Design review of the part built by this model. Coordinates are the model's own, in mm. A direction names the side the tool comes from. Coordinates: 2 decimals unless noted, no trailing zeros. Loops run counter-clockwise (first coordinate to the right, second up) from the corner with the lowest first, then second, coordinate; pieces in that order, holes last. Notation, with made-up numbers: (57.5, 30) -> (99.5, 30) arc R14 cw to (99.5, 47) -> close; hole circle Ø5 at (17.25, -38.75). An arc over 180 degrees is marked (long way). Use CSV: the item, a comma, the result in double quotes.
```python
from build123d import *

# Parameters (mm, degrees)
F0_R     = 12.7
F1_DEPTH = 25.4


with BuildPart() as f1:
    # F0 (on Front) → F1 (new body)
    with BuildSketch(Plane.XZ):
        with BuildLine():
            Line((16.9537905604, 25.4), (-42.3537905604, 25.4))
            ThreePointArc((-42.3537905604, 25.4), (-24.3932783182, 17.9605122421), (-16.9537905604, 0))
            ThreePointArc((-16.9537905604, 0), (-24.3932783182, -17.9605122421), (-42.3537905604, -25.4))
            Line((-42.3537905604, -25.4), (16.9537905604, -25.4))
            ThreePointArc((16.9537905604, -25.4), (34.9143028025, -17.9605122421), (42.3537905604, 0))
            ThreePointArc((42.3537905604, 0), (34.9143028025, 17.9605122421), (16.9537905604, 25.4))
        make_face()
        with Locations((16.9537905604, 0)):
            Circle(F0_R, mode=Mode.SUBTRACT)
        with BuildLine():
            Line((-42.3537905604, 14.224), (-42.3537905604, 25.4))
            ThreePointArc((-42.3537905604, 25.4), (-67.7537905604, 0), (-42.3537905604, -25.4))
            Line((-42.3537905604, -25.4), (-42.3537905604, -14.224))
            ThreePointArc((-42.3537905604, -14.224), (-56.5777905604, 0), (-42.3537905604, 14.224))
        make_face()
        with BuildLine():
            ThreePointArc((-16.9537905604, 0), (-24.3932783182, 17.9605122421), (-42.3537905604, 25.4))
            Line((-42.3537905604, 25.4), (-42.3537905604, 14.224))
            ThreePointArc((-42.3537905604, 14.224), (-33.8234800273, 11.3822659523), (-28.7016163276, 3.9925323692))
            Line((-28.7016163276, 3.9925323692), (-23.993383965, 3.9925323692))
            Line((-23.993383965, 3.9925323692), (-23.993383965, -3.9925323692))
            Line((-23.993383965, -3.9925323692), (-28.7016163276, -3.9925323692))
            ThreePointArc((-28.7016163276, -3.9925323692), (-33.8234800273, -11.3822659523), (-42.3537905604, -14.224))
            Line((-42.3537905604, -14.224), (-42.3537905604, -25.4))
            ThreePointArc((-42.3537905604, -25.4), (-24.3932783182, -17.9605122421), (-16.9537905604, 0))
        make_face()
    extrude(amount=F1_DEPTH)


solid = f1.part
```
Item 1: Add section A-A (y = -7.5). Give the boundary of the cut face in (x, z).
Checked values:
outline,"(-42.35, -25.4) -> (16.95, -25.4) arc R25.4 ccw to (16.95, 25.4) -> (-42.35, 25.4) arc R25.4 ccw to start; hole (-28.7, -3.99) -> (-23.99, -3.99) -> (-23.99, 3.99) -> (-28.7, 3.99) arc R14.22 ccw (long way) to start; hole circle Ø25.4 at (16.95, 0)"
Item 2: Machinability: for faces 1 (the face through (-26, -13, -3.993)), 2 (the face through (-13, -13, -25.4)), which of the approach directions +Z, -Z, +X, -X, +Y, -Y give a long, thin tool a straight path to every point of the face, cutting with its end or side? Answer none if there is none.
Checked values:
face 1,"+Y, -Y"
face 2,"-Z, +X, -X, +Y, -Y"
Item 3: Draft analysis for pull direction X (two halves, no side actions). For faces 3 (the face through (-23.993, -13, 0)), 4 (the face through (-12, -13, 25.4)), 5 (the face through (-67.748, -12.522, 0.559)), state which applies: pulls with the +X half, pulls with the -X half, needs draft (parallel to the pull), parting line crosses it, or undercut.
Checked values:
face 3,"undercut"
face 4,"needs draft"
face 5,"pulls with the -X half"
Item 4: To check wall thickness, follow line 1 along X through (y, z) = (-2.75, 10) (3 decimals); line 2 along Z through (x, y) = (-27.5, -10.75); line 3 along Z through (x, y) = (8.5, -8.75). State the ranges of each line that lie inside material, in increasing order.
Checked values:
line 1,"-65.702 to -52.469, -32.238 to 9.125, 24.783 to 40.302"
line 2,"-25.4 to -3.99, 3.99 to 25.4"
line 3,"-25.4 to -9.48, 9.48 to 25.4"
Item 5: Clearance check with flat-ended pins moving along their axes: pin 1 (6.5 mm diameter, centred on y = -7.5, z = 1.5, fed in from -X); pin 2 (3 mm diameter, centred on y = -12.5, z = 3, fed in from +X); pin 3 (3 mm diameter, centred on y = -16.5, z = -11, fed in from -X). State where each tip first meets the part, or that it passes through.
Checked values:
pin 1,"x = -67.75"
pin 2,"x = 42.31"
pin 3,"x = -65.91"
Item 6: Add section B-B (z = -18). Give the boundary of the cut face in (x, y).
Checked values:
outline,"(-60.27, -25.4) -> (34.87, -25.4) -> (34.87, 0) -> (-60.27, 0) -> close"
